```python
from build123d import *

# Parameters (mm, degrees)
SKETCH1_W           = 39
SKETCH1_H           = 31
SKETCH1_R           = 2.25
BOSS_EXTRUDE1_DEPTH = 8
FILLET2_R           = 1
CUT_EXTRUDE1_DEPTH  = 31


with BuildPart() as part:
    # Sketch1 → Boss-Extrude1 (new body)
    with BuildSketch(Plane(origin=(0, 0, 0), x_dir=(1, 0, 0), z_dir=(0, 1, 0))):
        with Locations((19.5, 15.5)):
            Rectangle(SKETCH1_W, SKETCH1_H)
        with Locations(Location((35.5, 23, 0), (0, 0, 270))):
            Circle(SKETCH1_R, mode=Mode.SUBTRACT)
        with Locations(Location((35.5, 8, 0), (0, 0, 90))):
            Circle(SKETCH1_R, mode=Mode.SUBTRACT)
        with Locations(Location((3.5, 23, 0), (0, 0, 90))):
            Circle(SKETCH1_R, mode=Mode.SUBTRACT)
        with Locations(Location((3.5, 8, 0), (0, 0, 270))):
            Circle(SKETCH1_R, mode=Mode.SUBTRACT)
    extrude(amount=BOSS_EXTRUDE1_DEPTH)

    # Fillet2
    fillet2_edges = [part.edges().sort_by_distance(p)[0] for p in [
        (39, 8, -15.5),
        (19.5, 8, -31),
        (0, 8, -15.5),
        (19.5, 8, 0),
        (0, 4, -31),
        (39, 4, -31),
        (39, 4, 0),
        (0, 4, 0),
    ]]
    fillet(fillet2_edges, radius=FILLET2_R)

    # Sketch2 → Cut-Extrude1 (cut)
    with BuildSketch(Plane.XY):
        with BuildLine():
            Line((10.33484861, 0), (-5.5, 0))
            Line((-5.5, 0), (-5.5, -10))
            Line((-5.5, -10), (44.5, -10))
            Line((44.5, -10), (44.5, 0))
            Line((44.5, 0), (28.66515139, 0))
            ThreePointArc((28.66515139, 0), (19.5, 4), (10.33484861, 0))
        make_face()
    extrude(amount=-CUT_EXTRUDE1_DEPTH, mode=Mode.SUBTRACT)


solid = part.part
```
Input: part model. Units: mm. Frame: model coordinates. Give positions to 0.01 mm unless a question says otherwise; leave off trailing zeros. Write each loop counter-clockwise with the first axis right and the second up, starting at its lowest first coordinate (ties: lowest second). Pieces come first, ordered by that corner, then holes. Notation, with made-up numbers: (50, 24.5) - (86, 24.5) arc R31 ccw to (86, 57.5) - close; hole circle Ø8 at (77, 48). An arc over 180 degrees is marked (long way). Write item = value, one per line. Start each with the question number.
1. Section query C-C, the plane y = 5. Output: boundary loops of the cut face in (x, z).
2. First-contact query: pin 1 Ø10 at (x, z) = (20, -9) entering from -Y (3 decimals). Flat tip, straight axial feed; report the tip coordinate or a pass-through.
3. Section query D-D, the plane z = -2. Output: boundary loops of the cut face in (x, y).
4. Ray query, L1, parallel to X at y = 4.5, z = -8; L2, parallel to X at y = 2.75, z = -8; L3, parallel to Z at x = 5, y = 7.25. Return the intervals inside material, ascending.
5. Section query A-A, the plane x = 3.5. Output: boundary loops of the cut face in (y, z), then the cut area to 3 significant figures.
6. Mould query, pull axis Z, two halves, no side actions, for faces 1 (the cylindrical face through (0.285, 3.549, -30.699)), 2 (the flat face through (19.2, 4.2, 0)), 3 (the cylindrical face through (33.27, 3.94, -7.71)), 4 (the flat face through (5, 0, -16)). Classes: released by +Z, released by -Z, zero draft, split by the parting line, or undercut.
7. Section query B-B, the plane z = -8. Output: boundary loops of the cut face in (x, y), then the cut area to 3 significant figures.
Check sheet entries:
q1.outline = (0, -30) arc R1 ccw to (1, -31) - (38, -31) arc R1 ccw to (39, -30) - (39, -1) arc R1 ccw to (38, 0) - (1, 0) arc R1 ccw to (0, -1) - close; hole circle Ø4.5 at (3.5, -23); hole circle Ø4.5 at (3.5, -8); hole circle Ø4.5 at (35.5, -23); hole circle Ø4.5 at (35.5, -8)
q2.pin_1 = 2.725
q3.outline = (0, 0) - (10.33, 0) arc R12.5 cw to (28.67, 0) - (39, 0) - (39, 7) arc R1 ccw to (38, 8) - (1, 8) arc R1 ccw to (0, 7) - close
q4.L1 = 0 to 1.25, 5.75 to 33.25, 37.75 to 39
q4.L2 = 0 to 1.25, 5.75 to 14.05, 24.95 to 33.25, 37.75 to 39
q4.L3 = -30.97 to -24.68, -21.32 to -9.68, -6.32 to -0.03
q5.outline = (0, -31) - (7, -31) arc R1 ccw to (8, -30) - (8, -25.25) - (0, -25.25) - close; (0, -20.75) - (8, -20.75) - (8, -10.25) - (0, -10.25) - close; (0, -5.75) - (8, -5.75) - (8, -1) arc R1 ccw to (7, 0) - (0, 0) - close
q5.area = 176 mm2
q6.face_1 = released by -Z
q6.face_2 = released by +Z
q6.face_3 = undercut
q6.face_4 = zero draft
q7.outline = (0, 0) - (1.25, 0) - (1.25, 8) - (1, 8) arc R1 ccw to (0, 7) - close; (5.75, 0) - (10.33, 0) arc R12.5 cw to (28.67, 0) - (33.25, 0) - (33.25, 8) - (5.75, 8) - close; (37.75, 0) - (39, 0) - (39, 7) arc R1 ccw to (38, 8) - (37.75, 8) - close
q7.area = 189 mm2
